Model file for the job. Use its own axes, mm. A direction names the side the tool comes from. Round coordinates to 2 decimals unless told otherwise and drop trailing zeros. Loops run counter-clockwise (first coordinate to the right, second up) from the corner with the lowest first, then second, coordinate; pieces in that order, holes last. Notation, with made-up numbers: (41.25, 27.5) - (51.25, 27.5) arc R34 ccw to (51.25, 61.5) - close; hole circle Ø8 at (46, 49). An arc over 180 degrees is marked (long way). Answer as a JSON object with one key per item and string values.
from build123d import *

# Parameters (mm, degrees)
BOSS_EXTRUDE1_DEPTH = 60
SKETCH2_W           = 80
SKETCH2_H           = 65
CUT_EXTRUDE1_DEPTH  = 60
CUT_EXTRUDE2_REACH  = 142
SKETCH3_R           = 1.5
CUT_EXTRUDE3_REACH  = 92
SKETCH4_R           = 5
SKETCH4_R_2         = 10
SKETCH4_R_3         = 2
FILLET1_R           = 2.5
FILLET3_R           = 2.5
FILLET4_R           = 2.5
FILLET5_R           = 2.5
FILLET6_R           = 2.5
SKETCH5_R           = 5
SKETCH5_R_2         = 2
CUT_EXTRUDE4_DEPTH  = 91
CUT_EXTRUDE5_REACH  = 92
SKETCH6_W           = 30
SKETCH6_H           = 10


with BuildPart() as part:
    # Sketch1 → Boss-Extrude1 (new body)
    with BuildSketch(Plane(origin=(0, 0, 0), x_dir=(0, 0, -1), z_dir=(1, 0, 0))):
        Polygon((0, 0), (0, -140), (-5, -140), (-5, -75), (-85, -75), (-85, -140), (-90, -140), (-90, 0), align=None)
    extrude(amount=-BOSS_EXTRUDE1_DEPTH)

    # Sketch2 → Cut-Extrude1 (cut)
    with BuildSketch(Plane(origin=(0, 0, 0), x_dir=(0, 0, -1), z_dir=(1, 0, 0))):
        with Locations((-45, -37.5)):
            Rectangle(SKETCH2_W, SKETCH2_H)
    extrude(amount=-CUT_EXTRUDE1_DEPTH, mode=Mode.SUBTRACT)

    # Sketch3 → Cut-Extrude2 (cut, up to next)
    with BuildSketch(Plane(origin=(0, 0, 0), x_dir=(1, 0, 0), z_dir=(0, 1, 0)), mode=Mode.PRIVATE) as cut_extrude2_sk1:
        with Locations((-24.5, -50.5)):
            Circle(SKETCH3_R)
    cut_extrude2_tool1 = extrude(cut_extrude2_sk1.sketch, amount=-CUT_EXTRUDE2_REACH, mode=Mode.PRIVATE) & part.part
    add(cut_extrude2_tool1.solids().sort_by_distance((-24.5, 0, 50.5))[0], mode=Mode.SUBTRACT)
    # Sketch3 → Cut-Extrude2 (cut, up to next)
    with BuildSketch(Plane(origin=(0, 0, 0), x_dir=(1, 0, 0), z_dir=(0, 1, 0)), mode=Mode.PRIVATE) as cut_extrude2_sk2:
        with Locations((-35.5, -50.5)):
            Circle(SKETCH3_R)
    cut_extrude2_tool2 = extrude(cut_extrude2_sk2.sketch, amount=-CUT_EXTRUDE2_REACH, mode=Mode.PRIVATE) & part.part
    add(cut_extrude2_tool2.solids().sort_by_distance((-35.5, 0, 50.5))[0], mode=Mode.SUBTRACT)
    # Sketch3 → Cut-Extrude2 (cut, up to next)
    with BuildSketch(Plane(origin=(0, 0, 0), x_dir=(1, 0, 0), z_dir=(0, 1, 0)), mode=Mode.PRIVATE) as cut_extrude2_sk3:
        with Locations((-35.5, -39.5)):
            Circle(SKETCH3_R)
    cut_extrude2_tool3 = extrude(cut_extrude2_sk3.sketch, amount=-CUT_EXTRUDE2_REACH, mode=Mode.PRIVATE) & part.part
    add(cut_extrude2_tool3.solids().sort_by_distance((-35.5, 0, 39.5))[0], mode=Mode.SUBTRACT)
    # Sketch3 → Cut-Extrude2 (cut, up to next)
    with BuildSketch(Plane(origin=(0, 0, 0), x_dir=(1, 0, 0), z_dir=(0, 1, 0)), mode=Mode.PRIVATE) as cut_extrude2_sk4:
        with Locations((-24.5, -39.5)):
            Circle(SKETCH3_R)
    cut_extrude2_tool4 = extrude(cut_extrude2_sk4.sketch, amount=-CUT_EXTRUDE2_REACH, mode=Mode.PRIVATE) & part.part
    add(cut_extrude2_tool4.solids().sort_by_distance((-24.5, 0, 39.5))[0], mode=Mode.SUBTRACT)
    # Sketch3 → Cut-Extrude2 (cut, up to next)
    with BuildSketch(Plane(origin=(0, 0, 0), x_dir=(1, 0, 0), z_dir=(0, 1, 0)), mode=Mode.PRIVATE) as cut_extrude2_sk5:
        with Locations((-12, -45)):
            Circle(SKETCH3_R)
    cut_extrude2_tool5 = extrude(cut_extrude2_sk5.sketch, amount=-CUT_EXTRUDE2_REACH, mode=Mode.PRIVATE) & part.part
    add(cut_extrude2_tool5.solids().sort_by_distance((-12, 0, 45))[0], mode=Mode.SUBTRACT)
    # Sketch3 → Cut-Extrude2 (cut, up to next)
    with BuildSketch(Plane(origin=(0, 0, 0), x_dir=(1, 0, 0), z_dir=(0, 1, 0)), mode=Mode.PRIVATE) as cut_extrude2_sk6:
        with Locations((-48, -45)):
            Circle(SKETCH3_R)
    cut_extrude2_tool6 = extrude(cut_extrude2_sk6.sketch, amount=-CUT_EXTRUDE2_REACH, mode=Mode.PRIVATE) & part.part
    add(cut_extrude2_tool6.solids().sort_by_distance((-48, 0, 45))[0], mode=Mode.SUBTRACT)

    # Sketch4 → Cut-Extrude3 (cut, up to next)
    with BuildSketch(Plane.XY, mode=Mode.PRIVATE) as cut_extrude3_sk1:
        with Locations((-30, -112)):
            Circle(SKETCH4_R)
    cut_extrude3_tool1 = extrude(cut_extrude3_sk1.sketch, amount=CUT_EXTRUDE3_REACH, mode=Mode.PRIVATE) & part.part
    add(cut_extrude3_tool1.solids().sort_by_distance((-30, -112, 0))[0], mode=Mode.SUBTRACT)
    # Sketch4 → Cut-Extrude3 (cut, up to next)
    with BuildSketch(Plane.XY, mode=Mode.PRIVATE) as cut_extrude3_sk2:
        with Locations((-30, -40)):
            Circle(SKETCH4_R_2)
    cut_extrude3_tool2 = extrude(cut_extrude3_sk2.sketch, amount=CUT_EXTRUDE3_REACH, mode=Mode.PRIVATE) & part.part
    add(cut_extrude3_tool2.solids().sort_by_distance((-30, -40, 0))[0], mode=Mode.SUBTRACT)
    # Sketch4 → Cut-Extrude3 (cut, up to next)
    with BuildSketch(Plane.XY, mode=Mode.PRIVATE) as cut_extrude3_sk3:
        with Locations((-5, -82)):
            Circle(SKETCH4_R_3)
    cut_extrude3_tool3 = extrude(cut_extrude3_sk3.sketch, amount=CUT_EXTRUDE3_REACH, mode=Mode.PRIVATE) & part.part
    add(cut_extrude3_tool3.solids().sort_by_distance((-5, -82, 0))[0], mode=Mode.SUBTRACT)
    # Sketch4 → Cut-Extrude3 (cut, up to next)
    with BuildSketch(Plane.XY, mode=Mode.PRIVATE) as cut_extrude3_sk4:
        with Locations((-55, -82)):
            Circle(SKETCH4_R_3)
    cut_extrude3_tool4 = extrude(cut_extrude3_sk4.sketch, amount=CUT_EXTRUDE3_REACH, mode=Mode.PRIVATE) & part.part
    add(cut_extrude3_tool4.solids().sort_by_distance((-55, -82, 0))[0], mode=Mode.SUBTRACT)
    # Sketch4 → Cut-Extrude3 (cut, up to next)
    with BuildSketch(Plane.XY, mode=Mode.PRIVATE) as cut_extrude3_sk5:
        with Locations((-14.5, -24.5)):
            Circle(SKETCH4_R_3)
    cut_extrude3_tool5 = extrude(cut_extrude3_sk5.sketch, amount=CUT_EXTRUDE3_REACH, mode=Mode.PRIVATE) & part.part
    add(cut_extrude3_tool5.solids().sort_by_distance((-14.5, -24.5, 0))[0], mode=Mode.SUBTRACT)
    # Sketch4 → Cut-Extrude3 (cut, up to next)
    with BuildSketch(Plane.XY, mode=Mode.PRIVATE) as cut_extrude3_sk6:
        with Locations((-45.5, -24.5)):
            Circle(SKETCH4_R_3)
    cut_extrude3_tool6 = extrude(cut_extrude3_sk6.sketch, amount=CUT_EXTRUDE3_REACH, mode=Mode.PRIVATE) & part.part
    add(cut_extrude3_tool6.solids().sort_by_distance((-45.5, -24.5, 0))[0], mode=Mode.SUBTRACT)
    # Sketch4 → Cut-Extrude3 (cut, up to next)
    with BuildSketch(Plane.XY, mode=Mode.PRIVATE) as cut_extrude3_sk7:
        with Locations((-45.5, -55.5)):
            Circle(SKETCH4_R_3)
    cut_extrude3_tool7 = extrude(cut_extrude3_sk7.sketch, amount=CUT_EXTRUDE3_REACH, mode=Mode.PRIVATE) & part.part
    add(cut_extrude3_tool7.solids().sort_by_distance((-45.5, -55.5, 0))[0], mode=Mode.SUBTRACT)
    # Sketch4 → Cut-Extrude3 (cut, up to next)
    with BuildSketch(Plane.XY, mode=Mode.PRIVATE) as cut_extrude3_sk8:
        with Locations((-14.5, -55.5)):
            Circle(SKETCH4_R_3)
    cut_extrude3_tool8 = extrude(cut_extrude3_sk8.sketch, amount=CUT_EXTRUDE3_REACH, mode=Mode.PRIVATE) & part.part
    add(cut_extrude3_tool8.solids().sort_by_distance((-14.5, -55.5, 0))[0], mode=Mode.SUBTRACT)

    # Fillet1
    fillet1_edges = [part.edges().sort_by_distance(p)[0] for p in [
        (-30, -75, 85),
    ]]
    fillet(fillet1_edges, radius=FILLET1_R)

    # Fillet3
    fillet3_edges = [part.edges().sort_by_distance(p)[0] for p in [
        (-30, -70, 85),
    ]]
    fillet(fillet3_edges, radius=FILLET3_R)

    # Fillet4
    fillet4_edges = [part.edges().sort_by_distance(p)[0] for p in [
        (-30, -70, 5),
    ]]
    fillet(fillet4_edges, radius=FILLET4_R)

    # Fillet5
    fillet5_edges = [part.edges().sort_by_distance(p)[0] for p in [
        (-30, -5, 5),
    ]]
    fillet(fillet5_edges, radius=FILLET5_R)

    # Fillet6
    fillet6_edges = [part.edges().sort_by_distance(p)[0] for p in [
        (-30, -5, 85),
    ]]
    fillet(fillet6_edges, radius=FILLET6_R)

    # Sketch5 → Cut-Extrude4 (cut, through all)
    with BuildSketch(Plane.XY.offset(90)):
        with Locations((-30, -112)):
            Circle(SKETCH5_R)
        with Locations((-12, -112)):
            Circle(SKETCH5_R_2)
        with Locations((-48, -112)):
            Circle(SKETCH5_R_2)
    extrude(amount=-CUT_EXTRUDE4_DEPTH, mode=Mode.SUBTRACT)

    # Sketch6 → Cut-Extrude5 (cut, up to next)
    with BuildSketch(Plane(origin=(0, 0, 0), x_dir=(-1, 0, 0), z_dir=(0, 0, -1)), mode=Mode.PRIVATE) as cut_extrude5_sk1:
        with Locations((15, -40)):
            Rectangle(SKETCH6_W, SKETCH6_H)
    cut_extrude5_tool1 = extrude(cut_extrude5_sk1.sketch, amount=-CUT_EXTRUDE5_REACH, mode=Mode.PRIVATE) & part.part
    add(cut_extrude5_tool1.solids().sort_by_distance((-15, -40, 0))[0], mode=Mode.SUBTRACT)


solid = part.part
1) Tool access for faces 4 (the cylindrical face through (-43.653, -25.266, 2.465)), 5 (the cylindrical face through (-12.325, -2.465, 46.464)), 6 (the flat face through (-30, -38, 85)), 7 (the cylindrical face through (-10.925, -110.314, 2.535)): list every direction of +Z, -Z, +X, -X, +Y, -Y with a clear straight run to the whole face (end or side of a thin tool).
Values follow:
{"face 4": "-Z", "face 5": "+Y", "face 6": "+X, -X", "face 7": "+Z, -Z"}
2) Two-plate mould, pull along Z, no slides. Class faces 1 (the cylindrical face through (-36.7, -2.5, 40.4)), 2 (the flat face through (-30, -71, 90)), 3 (the cylindrical face through (-34, -109, 2)): pulls with the +Z half, pulls with the -Z half, needs draft (parallel to the pull), parting line crosses it, or undercut.
Values follow:
{"face 1": "undercut", "face 2": "pulls with the +Z half", "face 3": "needs draft"}
3) Slice it at A-A on y = -55.5. List the corners of the cut face in (x, z), then the cut area to 3 significant figures.
Values follow:
{"outline": "(-60, 0) - (-47.5, 0) - (-47.5, 5) - (-60, 5) - close; (-60, 85) - (0, 85) - (0, 90) - (-60, 90) - close; (-43.5, 0) - (-16.5, 0) - (-16.5, 5) - (-43.5, 5) - close; (-12.5, 0) - (0, 0) - (0, 5) - (-12.5, 5) - close", "area": "560 mm²"}
4) Slice it at D-D on y = -112. Count the separate pieces of the cut face and the enclosed holes in it, then the cut area to 3 significant figures.
Values follow:
{"separate pieces": "8", "enclosed holes": "0", "area": "420 mm²"}
5) Slice it at B-B on z = 68.5. List the corners of the cut face in (x, y).
Values follow:
{"outline": "(-60, -75) - (0, -75) - (0, -70) - (-60, -70) - close; (-60, -5) - (0, -5) - (0, 0) - (-60, 0) - close"}
6) Drop flat-ended pins along their axis: P1, Ø10, axis at x = -37, z = 33, coming from the +Y side; P2, Ø1.8, axis at x = -35.5, z = 39.5, coming from the -Y side. Give the stop position or say it passes through.
Values follow:
{"P1": "y = 0", "P2": "y = -75"}
7) Slice it at C-C on x = -5. List the corners of the cut face in (y, z).
Values follow:
{"outline": "(-140, 0) - (-84, 0) - (-84, 5) - (-140, 5) - close; (-140, 85) - (-77.5, 85) arc R2.5 cw to (-75, 82.5) - (-75, 5) - (-80, 5) - (-80, 0) - (-45, 0) - (-45, 5) - (-67.5, 5) arc R2.5 cw to (-70, 7.5) - (-70, 82.5) arc R2.5 cw to (-67.5, 85) - (-7.5, 85) arc R2.5 cw to (-5, 82.5) - (-5, 7.5) arc R2.5 cw to (-7.5, 5) - (-35, 5) - (-35, 0) - (0, 0) - (0, 90) - (-140, 90) - close"}
8) Probe probe 1 along X at (y, z) = (-2.3, 39.5); probe 2 along X at (y, z) = (-82, 2); probe 3 along Y at (x, z) = (-5, 2.4). List the from-to ranges inside material, lowest first.
Values follow:
{"probe 1": "-60 to -37, -34 to -26, -23 to 0", "probe 2": "-60 to -57, -53 to -7, -3 to 0", "probe 3": "-140 to -84, -80 to -45, -35 to 0"}
